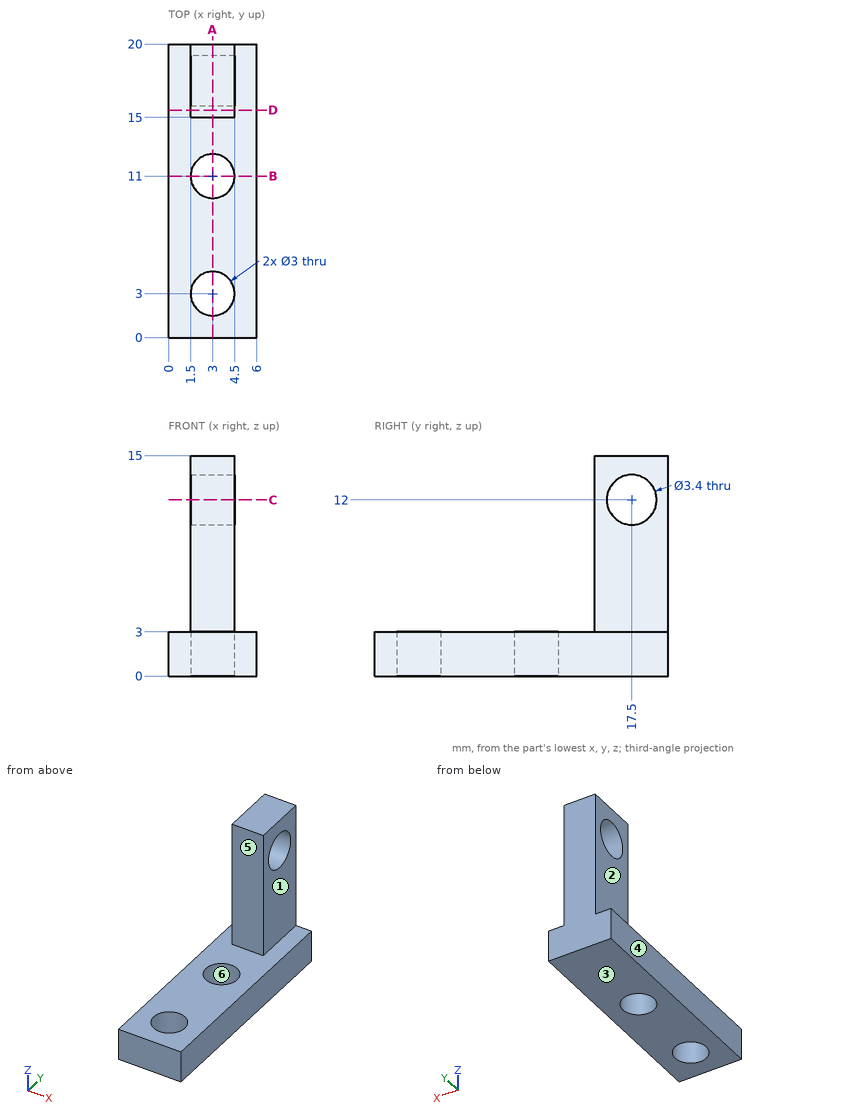
Verification items for this drawing (mm, ordinates from the low corner). A direction names the side the tool comes from. Coordinates: 2 decimals unless noted, no trailing zeros. Order: outer loops, then holes, each group sorted by start corner. A loop starts at its lowest first (then second) coordinate and runs counter-clockwise, first axis right, second up. Notation, with made-up numbers: (-13.75, 20) - (43.25, 20) arc R21 ccw to (43.25, 30) - close; hole circle Ø11 at (88.5, 66). An arc over 180 degrees is marked (long way). Answer in a Markdown table with one row per item. Add a question column.
1. Section check D-D (y = 15.5). Enter the section's corners in (x, z), plus the area to 3 significant figures.
2. Access from +Z, -Z, +X, -X, +Y, -Y to the whole of each face (thin tool, end or side, straight path). Record for the marked faces 1, 2 and 3.
3. Material ranges on L1, parallel to Y at x = 3, z = 1.8; L2, parallel to Z at x = 3.95, y = 17.5; L3, parallel to Z at x = 0.6, y = 7.25, recorded low to high. Write a range as [from, to].
4. Section check C-C (z = 12). Enter the section's corners in (x, y).
5. Section check A-A (x = 3). Enter the section's corners in (y, z).
6. Gauge pin test, flat ends, axial feed: pin 1 Ø2.5 at (y, z) = (18.5, 12) entering from +X; pin 2 Ø1.5 at (y, z) = (17, 4) entering from -X; pin 3 Ø3 at (x, y) = (2.5, 12) entering from +Z. Record the tip position at first contact, or that the pin passes through.
7. Section check B-B (y = 11). Enter the section's corners in (x, z).
8. Draft check along Y on the marked faces 4, 5 and 6. Enter one of: +Y half, -Y half, draft (parallel to the pull), parting line (faces both ways), or undercut.
Data:
| question | item | result |
|---|---|---|
| 1 | outline | (0, 0) - (6, 0) - (6, 3) - (4.5, 3) - (4.5, 15) - (1.5, 15) - (1.5, 3) - (0, 3) - close |
| 1 | area | 54.0 mm² |
| 2 | face 1 | +Z, +X, +Y, -Y |
| 2 | face 2 | +Z, -X, +Y, -Y |
| 2 | face 3 | -Z, +X, -X, +Y, -Y |
| 3 | L1 | y = [0, 1.5], [4.5, 9.5], [12.5, 20] |
| 3 | L2 | z = [0, 10.3], [13.7, 15] |
| 3 | L3 | z = [0, 3] |
| 4 | outline | (1.5, 15) - (4.5, 15) - (4.5, 15.8) - (1.5, 15.8) - close; (1.5, 19.2) - (4.5, 19.2) - (4.5, 20) - (1.5, 20) - close |
| 5 | outline | (0, 0) - (1.5, 0) - (1.5, 3) - (0, 3) - close; (4.5, 0) - (9.5, 0) - (9.5, 3) - (4.5, 3) - close; (12.5, 0) - (20, 0) - (20, 15) - (15, 15) - (15, 3) - (12.5, 3) - close; hole circle Ø3.4 at (17.5, 12) |
| 6 | pin 1 | stops at x = 4.5 |
| 6 | pin 2 | stops at x = 1.5 |
| 6 | pin 3 | stops at z = 3 |
| 7 | outline | (0, 0) - (1.5, 0) - (1.5, 3) - (0, 3) - close; (4.5, 0) - (6, 0) - (6, 3) - (4.5, 3) - close |
| 8 | face 4 | draft |
| 8 | face 5 | -Y half |
| 8 | face 6 | undercut |
